Could you check a few things on this drawing? It's one solid part, dimensions in mm from its lowest x, y, z. A direction names the side the tool comes from. Give positions to 0.01 mm unless a question says otherwise; leave off trailing zeros. Loops run counter-clockwise (first coordinate to the right, second up) from the corner with the lowest first, then second, coordinate; pieces in that order, holes last. Notation, with made-up numbers: (34.25, 89.5) -> (76.25, 89.5) arc R15 cw to (76.25, 102.5) -> close; hole circle Ø8 at (37.25, -24). An arc over 180 degrees is marked (long way). Use CSV: the item, a comma, the result in double quotes.
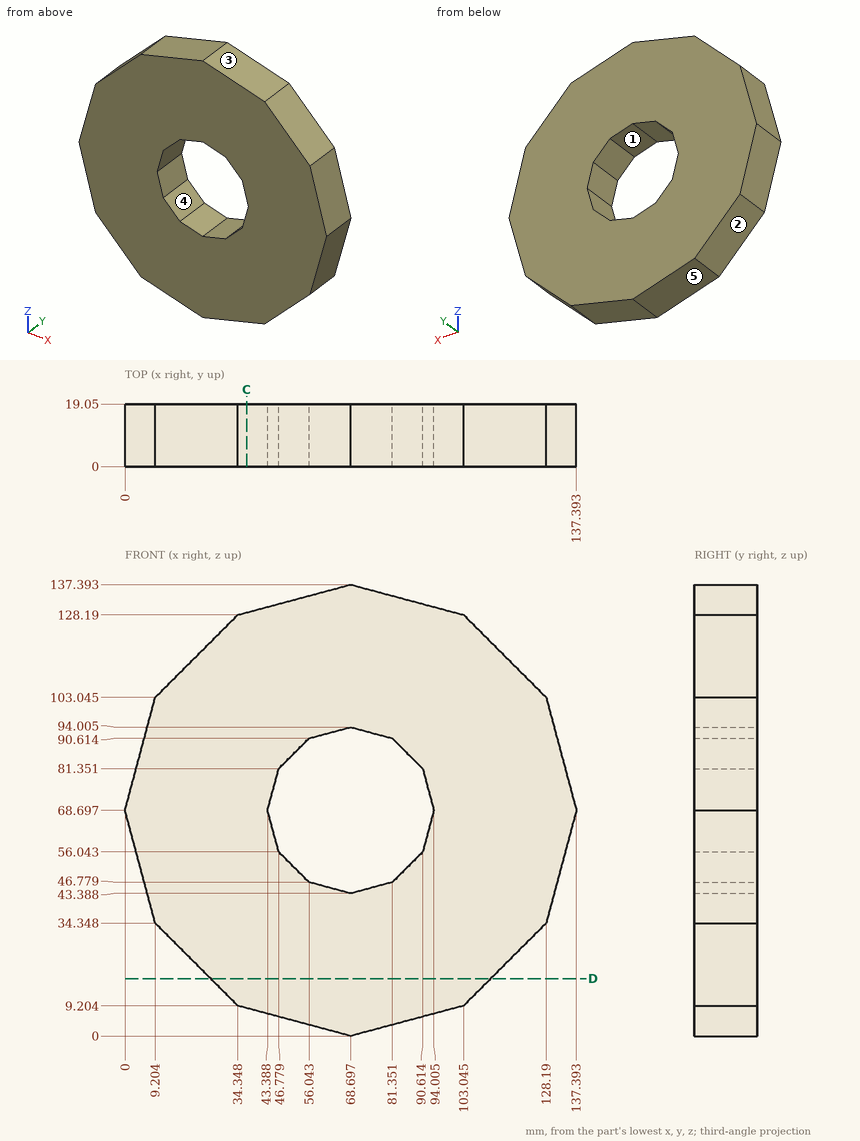
(1) If we section it at D-D, the plane z = 17.5: Write out the boundary of the cut face in (x, y).
Answer sheet:
outline,"(26.05, 0) -> (111.34, 0) -> (111.34, 19.05) -> (26.05, 19.05) -> close"
(2) Will these pins go through, and if not, where does the flat tip stop? pin 1 Ø2 at (y, z) = (5, 101) entering from +X (1 decimal); pin 2 Ø8 at (y, z) = (14.5, 78) entering from -X; pin 3 Ø4 at (y, z) = (13, 20) entering from +X.
Answer sheet:
pin 1,"stops at x = 129"
pin 2,"stops at x = 1.42"
pin 3,"stops at x = 115.84"
(3) Which directions (+Z, -Z, +X, -X, +Y, -Y) give clear straight access to the entire face, cutting with the end or side of a thin tool? Please do the marked faces 1 and 2.
Answer sheet:
face 1,"+Y, -Y"
face 2,"-Z, -X, +Y, -Y"
(4) We'd pull the mould along X, two halves only. Please class the marked faces 3, 4 and 5: released by +X, released by -X, zero draft, split by the parting line, or undercut.
Answer sheet:
face 3,"released by +X"
face 4,"undercut"
face 5,"released by -X"
(5) If we section it at C-C, the plane x = 37: Write out the boundary of the cut face in (y, z), then the cut area to 3 significant figures.
Answer sheet:
outline,"(0, 8.49) -> (19.05, 8.49) -> (19.05, 128.9) -> (0, 128.9) -> close"
area,"2,290 mm2"
(6) If I drill on L1, parallel to Z at x = 88, y = 4.75 (1 decimal); L2, parallel to Z at x = 56.5, y = 6.25 (1 decimal); L3, parallel to X at y = 7.25, z = 70.5, over which ranges is the centre line in solid material (lowest first)? Write a range as from..to.
Answer sheet:
L1,"z = 5.2..53.4, 84..132.2"
L2,"z = 3.3..46.7, 90.7..134.1"
L3,"x = 0.48..43.87, 93.52..136.91"
